Input: part model. Units: mm. Frame: model coordinates. Face numbers are marked on the shaded views. A direction names the side the tool comes from. Give positions to 0.01 mm unless a question says otherwise; leave off trailing zeros. Loops run counter-clockwise (first coordinate to the right, second up) from the corner with the lowest first, then second, coordinate; pieces in that order, holes last. Notation, with made-up numbers: (35.5, 10) - (50.5, 10) arc R28 cw to (50.5, 29) - close; hole circle Ø3 at (18.25, 33). An arc over 180 degrees is marked (long way). Answer as a JSON object with one key per item and string values. Group by question number.
(1) Section query B-B (x = 0). Return loops of the section in (y, z).
(2) Section query D-D (y = 39). Return loops of the section in (x, z), plus the area to 3 significant figures.
(3) Access query for the marked faces 1 and 2. Directions: +Z, -Z, +X, -X, +Y, -Y. A direction counts if a zero-diameter tool reaches every point of the face in a straight line with its end or side. Return the directions, or none.
(4) Pin query (flat end, axial travel): P1, Ø3, axis at x = 58.5, z = -2.5, coming from the +Y side; P2, Ø2, axis at y = 12.5, z = -15, coming from the +X side; P3, Ø8, axis at y = 3.5, z = 75, coming from the +X side. Return the tip coordinate at first contact, or that it passes through.
(5) Material intervals for L1, parallel to X at y = 12, z = -9; L2, parallel to Y at x = -159, z = 70.5; L3, parallel to Z at x = -32, y = 7, sorted ascending.
(6) Section query C-C (z = 65). Return loops of the section in (x, y), plus the area to 3 significant figures.
(7) Section query A-A (y = 15). Return loops of the section in (x, z), plus the area to 3 significant figures.
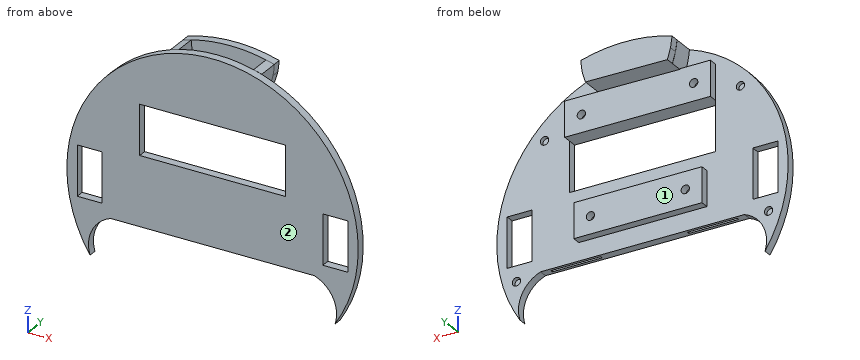
```python
from build123d import *

# Parameters (mm, degrees)
BASEDIA_R           = 175
BOSS_EXTRUDE1_DEPTH = 10
SKETCH2_W           = 175
SKETCH2_H           = 60
CUT_EXTRUDE3_DEPTH  = 10
CUT_EXTRUDE5_START  = -10
SKETCH5_W           = 30
SKETCH5_H           = 60
CUT_EXTRUDE5_DEPTH  = 10
BOSS_EXTRUDE2_DEPTH = 25
SKETCH8_W           = 175
SKETCH8_H           = 42.297309852
SKETCH8_R           = 5
BOSS_EXTRUDE3_DEPTH = 10
SKETCH9_W           = 154
SKETCH9_H           = 42
SKETCH9_R           = 5
BOSS_EXTRUDE4_DEPTH = 10
SKETCH10_R          = 5
CUT_EXTRUDE6_DEPTH  = 5
SKETCH11_W          = 60
SKETCH11_H          = 3
CUT_EXTRUDE7_DEPTH  = 10
BOSS_EXTRUDE5_DEPTH = 10


with BuildPart() as part:
    # basedia → Boss-Extrude1 (new body)
    with BuildSketch(Plane(origin=(0, 0, 0), x_dir=(1, 0, 0), z_dir=(0, 1, 0))):
        with Locations(Location((0, 0, 0), (0, 0, 270))):
            Circle(BASEDIA_R)
    extrude(amount=BOSS_EXTRUDE1_DEPTH)

    # Sketch2 → Cut-Extrude3 (cut)
    with BuildSketch(Plane(origin=(0, 0, 0), x_dir=(1, 0, 0), z_dir=(0, 1, 0))):
        with Locations((0, -68.076429651)):
            Rectangle(SKETCH2_W, SKETCH2_H)
    extrude(amount=CUT_EXTRUDE3_DEPTH, mode=Mode.SUBTRACT)

    # Sketch5 → Cut-Extrude5 (cut)
    with BuildSketch(Plane(origin=(0, 10, 0), x_dir=(1, 0, 0), z_dir=(0, 1, 0)).offset(CUT_EXTRUDE5_START)):
        with BuildLine():
            Line((-122.466018466, 45), (122.466018466, 45))
            ThreePointArc((122.466018466, 45), (144.830685243, 64.836208714), (147.204111427, 94.63587892))
            ThreePointArc((147.204111427, 94.63587892), (0, 175), (-147.204111427, 94.63587892))
            ThreePointArc((-147.204111427, 94.63587892), (-144.830685243, 64.836208714), (-122.466018466, 45))
        make_face()
        with Locations((-147.5, 0)):
            Rectangle(SKETCH5_W, SKETCH5_H)
        with Locations((147.5, 0)):
            Rectangle(SKETCH5_W, SKETCH5_H)
    extrude(amount=CUT_EXTRUDE5_DEPTH, mode=Mode.SUBTRACT)

    # Sketch7 → Boss-Extrude2 (add)
    with BuildSketch(Plane(origin=(0, 10, 0), x_dir=(1, 0, 0), z_dir=(0, 1, 0))):
        with BuildLine():
            Line((-43.56510526, -149.674915049), (40.559642833, -150.319684554))
            ThreePointArc((40.559642833, -150.319684554), (42.642034938, -159.836675376), (43.310651761, -169.555853464))
            Line((43.310651761, -169.555853464), (53.279307238, -167.030646365))
            ThreePointArc((53.279307238, -167.030646365), (51.661940371, -153.449452713), (47.650653713, -140.373739503))
            Line((47.650653713, -140.373739503), (-50.823489188, -139.61898985))
            ThreePointArc((-50.823489188, -139.61898985), (-54.540052947, -152.439162742), (-56.427487426, -165.65306717))
            Line((-56.427487426, -165.65306717), (-46.575152469, -168.40822556))
            ThreePointArc((-46.575152469, -168.40822556), (-45.593073163, -158.957544204), (-43.56510526, -149.674915049))
        make_face()
    extrude(amount=BOSS_EXTRUDE2_DEPTH)

    # Sketch8 → Boss-Extrude3 (add)
    with BuildSketch(Plane(origin=(0, 10, 0), x_dir=(1, 0, 0), z_dir=(0, 1, 0))):
        with Locations((0, -119.225084577)):
            Rectangle(SKETCH8_W, SKETCH8_H)
        with Locations(Location((-67.5, -119.225084577, 0), (0, 0, 270))):
            Circle(SKETCH8_R, mode=Mode.SUBTRACT)
        with Locations(Location((67.5, -119.225084577, 0), (0, 0, 270))):
            Circle(SKETCH8_R, mode=Mode.SUBTRACT)
    extrude(amount=BOSS_EXTRUDE3_DEPTH)

    # Sketch9 → Boss-Extrude4 (add)
    with BuildSketch(Plane(origin=(0, 10, 0), x_dir=(1, 0, 0), z_dir=(0, 1, 0))):
        with Locations((-0.423800225, 2.37885536)):
            Rectangle(SKETCH9_W, SKETCH9_H)
        with Locations(Location((-57.423800225, 2.37885536, 0), (0, 0, 270))):
            Circle(SKETCH9_R, mode=Mode.SUBTRACT)
        with Locations(Location((56.576199775, 2.37885536, 0), (0, 0, 270))):
            Circle(SKETCH9_R, mode=Mode.SUBTRACT)
    extrude(amount=BOSS_EXTRUDE4_DEPTH)

    # Sketch10 → Cut-Extrude6 (cut)
    with BuildSketch(Plane(origin=(0, 10, 0), x_dir=(1, 0, 0), z_dir=(0, 1, 0))):
        with Locations(Location((-117.665653332, -106.704862813, 0), (0, 0, 270))):
            Circle(SKETCH10_R)
        with Locations(Location((-151.426262726, 48.693236313, 0), (0, 0, 270))):
            Circle(SKETCH10_R)
        with Locations(Location((151.426262726, 48.693236313, 0), (0, 0, 90))):
            Circle(SKETCH10_R)
        with Locations(Location((117.665653332, -106.704862813, 0), (0, 0, 90))):
            Circle(SKETCH10_R)
    extrude(amount=-CUT_EXTRUDE6_DEPTH, mode=Mode.SUBTRACT)

    # Sketch11 → Cut-Extrude7 (cut)
    with BuildSketch(Plane(origin=(0, 0, -45), x_dir=(-1, 0, 0), z_dir=(0, 0, -1))):
        with Locations((-82.041456067, 5.240211955)):
            Rectangle(SKETCH11_W, SKETCH11_H)
        with Locations((82.041456067, 5.240211955)):
            Rectangle(SKETCH11_W, SKETCH11_H)
    extrude(amount=-CUT_EXTRUDE7_DEPTH, mode=Mode.SUBTRACT)

    # Sketch12 → Boss-Extrude5 (add)
    with BuildSketch(Plane(origin=(0, 35, 0), x_dir=(1, 0, 0), z_dir=(0, 1, 0))):
        with BuildLine():
            Line((-50.823489188, -139.61898985), (47.650653713, -140.373739503))
            Line((47.650653713, -140.373739503), (51.661940371, -153.449452713))
            Line((51.661940371, -153.449452713), (53.279307238, -167.030646365))
            ThreePointArc((53.279307238, -167.030646365), (-1.675350263, -174.405951078), (-56.427487426, -165.65306717))
            Line((-56.427487426, -165.65306717), (-54.540052947, -152.439162742))
            Line((-54.540052947, -152.439162742), (-50.823489188, -139.61898985))
        make_face()
    extrude(amount=BOSS_EXTRUDE5_DEPTH)


solid = part.part
```
Recorded:
{
 "1": {"outline": "(0, -45) - (10, -45) - (10, -23.38) - (20, -23.38) - (20, 18.62) - (10, 18.62) - (10, 38.08) - (0, 38.08) - close; (0, 98.08) - (20, 98.08) - (20, 140.01) - (45, 140.01) - (45, 174.42) - (35, 174.42) - (35, 150.01) - (10, 150.01) - (10, 175) - (0, 175) - close"},
 "2": {"outline": "(-56.43, 165.65) - (-54.54, 152.44) - (-50.82, 139.62) - (47.65, 140.37) - (51.66, 153.45) - (53.28, 167.03) arc R190.61 ccw to start", "area": "3,360 mm^2"},
 "3": {"face 1": "-Z, +X, -X, +Y", "face 2": "+Z, -Z, +X, -X, -Y"},
 "4": {"P1": "stops at y = 10", "P2": "stops at x = 76.58", "P3": "stops at x = 159.95"},
 "5": {"L1": "x = -77.42 to 76.58", "L2": "y = 0 to 10", "L3": "z = -45 to 38.08, 98.08 to 172.05"},
 "6": {"outline": "(-162.48, 0) - (-87.5, 0) - (-87.5, 10) - (-162.48, 10) - close; (87.5, 0) - (162.48, 0) - (162.48, 10) - (87.5, 10) - close", "area": "1,500 mm^2"},
 "7": {"outline": "(-87.5, 98.08) - (87.5, 98.08) - (87.5, 140.37) - (47.65, 140.37) arc R76.46 ccw to (53.28, 167.03) - (43.31, 169.56) arc R66.46 cw to (40.56, 150.32) - (-43.57, 149.67) arc R85.23 cw to (-46.58, 168.41) - (-56.43, 165.65) arc R95.23 ccw to (-51.1, 140.37) - (-87.5, 140.37) - close; (-77.42, -23.38) - (76.58, -23.38) - (76.58, 18.62) - (-77.42, 18.62) - close; hole circle Ø10 at (-67.5, 119.23); hole circle Ø10 at (-57.42, -2.38); hole circle Ø10 at (56.58, -2.38); hole circle Ø10 at (67.5, 119.23)", "area": "14,900 mm^2"}
}
